Build history of the part. All positions in model axes, mm. Round coordinates to 2 decimals unless told otherwise and drop trailing zeros. Write each loop counter-clockwise with the first axis right and the second up, starting at its lowest first coordinate (ties: lowest second). Pieces come first, ordered by that corner, then holes. Notation, with made-up numbers: M 13.25,-23.75 L 51.25,-23.75 A4 cw 51.25,-17.75 Z; hole C 43.25,87.5 d11. An arc over 180 degrees is marked long. Write item = value, one per line.
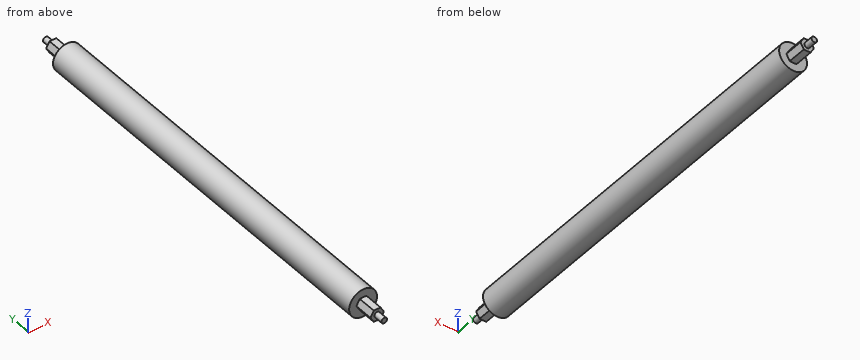
from build123d import *

# Parameters (mm, degrees)
SKETCH2_R           = 7.5
BOSS_EXTRUDE1_DEPTH = 240
CUT_EXTRUDE1_START  = -15
SKETCH3_R           = 7.5
SKETCH3_R_2         = 1.5
CUT_EXTRUDE1_DEPTH  = 15
BOSS_EXTRUDE2_DEPTH = 10


with BuildPart() as part:
    # Sketch2 → Boss-Extrude1 (new body)
    with BuildSketch(Plane(origin=(0, 0, 0), x_dir=(1, 0, 0), z_dir=(0, 1, 0))):
        with Locations(Location((0, 0, 0), (0, 0, 270))):
            Circle(SKETCH2_R)
    extrude(amount=BOSS_EXTRUDE1_DEPTH)

    # Sketch3 → Cut-Extrude1 (cut)
    with BuildSketch(Plane(origin=(0, 240, 0), x_dir=(1, 0, 0), z_dir=(0, 1, 0)).offset(CUT_EXTRUDE1_START)):
        with Locations(Location((0, 0, 0), (0, 0, 270))):
            Circle(SKETCH3_R)
        with Locations(Location((0, 0, 0), (0, 0, 270))):
            Circle(SKETCH3_R_2, mode=Mode.SUBTRACT)
    cut_extrude1 = extrude(amount=CUT_EXTRUDE1_DEPTH, mode=Mode.SUBTRACT)

    # Sketch4 → Boss-Extrude2 (add)
    with BuildSketch(Plane(origin=(0, 225, 0), x_dir=(1, 0, 0), z_dir=(0, 1, 0))):
        Polygon((-1.8, 3.117691454), (1.8, 3.117691454), (3.6, 0), (1.8, -3.117691454), (-1.8, -3.117691454), (-3.6, 0), align=None)
    boss_extrude2 = extrude(amount=BOSS_EXTRUDE2_DEPTH)

    # Mirror1: Cut-Extrude1, Boss-Extrude2 across plane
    add(cut_extrude1.mirror(Plane.ZX.offset(120)), mode=Mode.SUBTRACT)
    add(boss_extrude2.mirror(Plane.ZX.offset(120)))


solid = part.part
1. Flat gauge pins, fed straight in: pin 1 (1.5 mm diameter, centred on x = -5, z = -2, fed in from -Y); pin 2 (1.1 mm diameter, centred on x = -1, y = 8.5, fed in from +Z); pin 3 (3 mm diameter, centred on x = 2.5, y = 88.5, fed in from +Z). Where does each tip first touch, or does it go through?
Responses:
pin_1 = 15
pin_2 = 3.12
pin_3 = 7.43
2. Band-saw the part on A-A (y = 203). List the corners of the cut face in (x, z).
Responses:
outline = C 0,0 d15
3. Probe probe 1 along Y at (x, z) = (3.5, -6.25); probe 2 along X at (y, z) = (74.5, 0.75); probe 3 along Z at (x, y) = (0.25, 206). List the from-to ranges inside material, lowest first.
Responses:
probe_1 = 15 to 225
probe_2 = -7.46 to 7.46
probe_3 = -7.5 to 7.5
